from build123d import *
from build123d.topology import SkipClean

# Parameters (mm, degrees)
SKETCH1_R             = 100
BOSS_EXTRUDE1_DEPTH   = 10
SKETCH2_R             = 32.5
CUT_EXTRUDE1_DEPTH    = 250
LPATTERN5_START       = -190
LPATTERN5_OUTLINE_R   = 100
LPATTERN5_OUTLINE_R_2 = 32.5
LPATTERN5_DEPTH       = 190


# Read off the part's stored shape, not the designer's step: LPattern5
with BuildPart() as part:
    # Sketch1 → Boss-Extrude1 (new body)
    with BuildSketch(Plane(origin=(0, 0, 0), x_dir=(0, 0, -1), z_dir=(1, 0, 0))):
        Circle(SKETCH1_R)
    extrude(amount=BOSS_EXTRUDE1_DEPTH)

    # Sketch2 → Cut-Extrude1 (cut)
    with BuildSketch(Plane(origin=(10, 0, 0), x_dir=(0, 0, -1), z_dir=(1, 0, 0))):
        Circle(SKETCH2_R)
        Polygon((1.047809143, 84.212465352), (2.321864858, 76.712465352), (42.321864858, 79.227207296), (46.796605305, 83.651032908), (43.720430917, 86.727207296), (41.047809143, 86.727207296), align=None)
        Polygon((-1.047809143, 84.212465352), (-2.321864858, 76.712465352), (-42.321864858, 79.227207296), (-46.796605305, 83.651032908), (-43.720430917, 86.727207296), (-41.047809143, 86.727207296), align=None)
        Polygon((84.212465352, 1.047809143), (76.712465352, 2.321864858), (79.227207296, 42.321864858), (83.651032908, 46.796605305), (86.727207296, 43.720430917), (86.727207296, 41.047809143), align=None)
        Polygon((84.212465352, -1.047809143), (86.727207296, -41.047809143), (86.727207296, -43.720430917), (83.651032908, -46.796605305), (79.227207296, -42.321864858), (76.712465352, -2.321864858), align=None)
        Polygon((1.047809143, -84.212465352), (2.321864858, -76.712465352), (42.321864858, -79.227207296), (46.796605305, -83.651032908), (43.720430917, -86.727207296), (41.047809143, -86.727207296), align=None)
        Polygon((-1.047809143, -84.212465352), (-41.047809143, -86.727207296), (-43.720430917, -86.727207296), (-46.796605305, -83.651032908), (-42.321864858, -79.227207296), (-2.321864858, -76.712465352), align=None)
        Polygon((-84.212465352, -1.047809143), (-76.712465352, -2.321864858), (-79.227207296, -42.321864858), (-83.651032908, -46.796605305), (-86.727207296, -43.720430917), (-86.727207296, -41.047809143), align=None)
        Polygon((-84.212465352, 1.047809143), (-86.727207296, 41.047809143), (-86.727207296, 43.720430917), (-83.651032908, 46.796605305), (-79.227207296, 42.321864858), (-76.712465352, 2.321864858), align=None)
    extrude(amount=-CUT_EXTRUDE1_DEPTH, mode=Mode.SUBTRACT)

    # LPattern5 outline → LPattern5 (add)
    with SkipClean():  # the faces are left unmerged after this step: merging them gives an invalid solid
        with BuildSketch(Plane.YZ.offset(LPATTERN5_START)):
            Circle(LPATTERN5_OUTLINE_R)
            Polygon((-43.720430917, -86.727207296), (-46.796605305, -83.651032908), (-42.321864858, -79.227207296), (-2.321864858, -76.712465352), (-1.047809143, -84.212465352), (-41.047809143, -86.727207296), align=None, mode=Mode.SUBTRACT)
            Polygon((-86.727207296, -43.720430917), (-86.727207296, -41.047809143), (-84.212465352, -1.047809143), (-76.712465352, -2.321864858), (-79.227207296, -42.321864858), (-83.651032908, -46.796605305), align=None, mode=Mode.SUBTRACT)
            Polygon((43.720430917, -86.727207296), (41.047809143, -86.727207296), (1.047809143, -84.212465352), (2.321864858, -76.712465352), (42.321864858, -79.227207296), (46.796605305, -83.651032908), align=None, mode=Mode.SUBTRACT)
            Polygon((86.727207296, -41.047809143), (86.727207296, -43.720430917), (83.651032908, -46.796605305), (79.227207296, -42.321864858), (76.712465352, -2.321864858), (84.212465352, -1.047809143), align=None, mode=Mode.SUBTRACT)
            Polygon((-86.727207296, 43.720430917), (-83.651032908, 46.796605305), (-79.227207296, 42.321864858), (-76.712465352, 2.321864858), (-84.212465352, 1.047809143), (-86.727207296, 41.047809143), align=None, mode=Mode.SUBTRACT)
            Polygon((-43.720430917, 86.727207296), (-41.047809143, 86.727207296), (-1.047809143, 84.212465352), (-2.321864858, 76.712465352), (-42.321864858, 79.227207296), (-46.796605305, 83.651032908), align=None, mode=Mode.SUBTRACT)
            Circle(LPATTERN5_OUTLINE_R_2, mode=Mode.SUBTRACT)
            Polygon((86.727207296, 41.047809143), (84.212465352, 1.047809143), (76.712465352, 2.321864858), (79.227207296, 42.321864858), (83.651032908, 46.796605305), (86.727207296, 43.720430917), align=None, mode=Mode.SUBTRACT)
            Polygon((43.720430917, 86.727207296), (46.796605305, 83.651032908), (42.321864858, 79.227207296), (2.321864858, 76.712465352), (1.047809143, 84.212465352), (41.047809143, 86.727207296), align=None, mode=Mode.SUBTRACT)
        extrude(amount=LPATTERN5_DEPTH)


solid = part.part
Geometry: final body of the model. Coordinates: model frame, mm. A direction names the side the tool comes from. Coordinates: 2 decimals unless noted, no trailing zeros. Loops run counter-clockwise (first coordinate to the right, second up) from the corner with the lowest first, then second, coordinate; pieces in that order, holes last. Notation, with made-up numbers: M -21.75,28.25 L -1.75,28.25 A20 ccw -1.75,58.25 Z; hole C 18,49.5 d4. An arc over 180 degrees is marked long. One line per item, written item: value. Start each with the question number.
1) Cut plane B-B (x = -102). Count the separate pieces of the cut face and the enclosed holes in it, then the cut area to 3 significant figures.
2) Reachability of faces 3 (the flat face through (10, 24, 24)), 4 (the flat face through (-91.4, 21.328, -85.487)) from +Z, -Z, +X, -X, +Y, -Y: full face, straight path, thin tool, end or side. Return the list, or none.
3) Cut plane A-A (z = 21). Return loops of the section in (x, y), then the cut area to 3 significant figures.
4) Cut plane C-C (z = 62.5). Return loops of the section in (x, y), then the cut area to 3 significant figures.
5) Material intervals for L1, parallel to Y at x = -51, z = 0; L2, parallel to Y at x = -178, z = 34, sorted ascending. Write a range as from..to.
6) Pin query (flat end, axial travel): P1, Ø0.8, axis at x = -65.5, y = 43, coming from the -Z side; P2, Ø2, axis at x = -83, y = 42, coming from the +Z side; P3, Ø2, axis at x = -115.5, z = -42.5, coming from the -Y side. Return the tip coordinate at first contact, or that it passes through.
7) Draft query along Y for faces 1 (the flat face through (-190, -24, 24)), 2 (the flat face through (-91.4, 1.676, -80.515)). Return one class per face: released by +Y, released by -Y, zero draft, split by the parting line, or undercut.
Evaluation:
1. separate pieces: 1
1. enclosed holes: 9
1. area: 25,500 mm^2
2. face 3: +Z, -Z, +X, +Y, -Y
2. face 4: +X, -X
3. outline: M -190,-97.77 L 10,-97.77 L 10,-85.47 L -190,-85.47 Z; M -190,-77.89 L 10,-77.89 L 10,-24.8 L -190,-24.8 Z; M -190,24.8 L 10,24.8 L 10,77.89 L -190,77.89 Z; M -190,85.47 L 10,85.47 L 10,97.77 L -190,97.77 Z
3. area: 26,200 mm^2
4. outline: M -190,-78.06 L 10,-78.06 L 10,78.06 L -190,78.06 Z
4. area: 31,200 mm^2
5. L1: -100..-32.5, 32.5..100
5. L2: -94.04..-86.28, -78.7..78.7, 86.28..94.04
6. P1: z = -90.47
6. P2: z = 91.21
6. P3: y = -90.98
7. face 1: zero draft
7. face 2: undercut
